Check sheet for the modelled part. Datum: model origin and axes. Units: mm. Give positions to 0.01 mm unless a question says otherwise; leave off trailing zeros. Write each loop counter-clockwise with the first axis right and the second up, starting at its lowest first coordinate (ties: lowest second). Pieces come first, ordered by that corner, then holes. Notation, with made-up numbers: (81.5, 11) -> (137.5, 11) arc R7 ccw to (137.5, 23) -> close; hole circle Ø9 at (70, 79). An arc over 180 degrees is marked (long way). Answer as a JSON object with one key per item and string values.
from build123d import *

# Parameters (mm, degrees)
CHAMFER1_SIZE = 0.2
CHAMFER2_SIZE = 0.2
CHAMFER3_SIZE = 0.5
CHAMFER4_SIZE = 0.5
FILLET2_R     = 0.2


with BuildPart() as part:
    # Sketch1 → Revolve1 (revolve)
    with BuildSketch(Plane.XY, mode=Mode.PRIVATE) as revolve1_sk:
        Polygon((0, 0), (117, 0), (117, 1.5), (112, 1.5), (112, 3), (3, 3), (3, 2.5), (0, 2.5), align=None)
    revolve(revolve1_sk.sketch.rotate(Axis((0, 0, 0), (1, 0, 0)), 90), axis=Axis((0, 0, 0), (1, 0, 0)))

    # Chamfer1
    chamfer1_edges = [part.edges().sort_by_distance(p)[0] for p in [
        (112, 0, -3),
    ]]
    chamfer(chamfer1_edges, length=CHAMFER1_SIZE)

    # Chamfer2
    chamfer2_edges = [part.edges().sort_by_distance(p)[0] for p in [
        (3, 0, -3),
    ]]
    chamfer(chamfer2_edges, length=CHAMFER2_SIZE)

    # Chamfer3
    chamfer3_edges = [part.edges().sort_by_distance(p)[0] for p in [
        (0, 0, -2.5),
    ]]
    chamfer(chamfer3_edges, length=CHAMFER3_SIZE)

    # Chamfer4
    chamfer4_edges = [part.edges().sort_by_distance(p)[0] for p in [
        (117, 0, -1.5),
    ]]
    chamfer(chamfer4_edges, length=CHAMFER4_SIZE)

    # Fillet2
    fillet2_edges = [part.edges().sort_by_distance(p)[0] for p in [
        (112, 0, -1.5),
    ]]
    fillet(fillet2_edges, radius=FILLET2_R)


solid = part.part
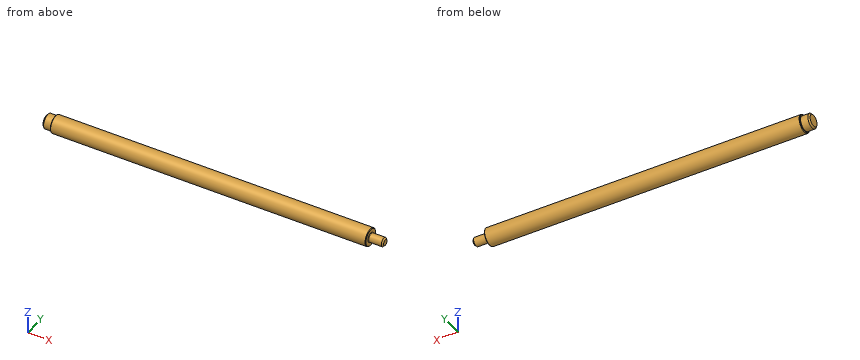
1. Sectioned sample at A-A, the plane z = 0. Enter the section's corners in (x, y).
Determined:
{"outline": "(0, -2) -> (0.5, -2.5) -> (3, -2.5) -> (3, -2.8) -> (3.2, -3) -> (111.8, -3) -> (112, -2.8) -> (112, -1.7) arc R0.2 cw to (112.2, -1.5) -> (116.5, -1.5) -> (117, -1) -> (117, 1) -> (116.5, 1.5) -> (112.2, 1.5) arc R0.2 cw to (112, 1.7) -> (112, 2.8) -> (111.8, 3) -> (3.2, 3) -> (3, 2.8) -> (3, 2.5) -> (0.5, 2.5) -> (0, 2) -> close"}
2. Sectioned sample at C-C, the plane x = 12.5. Enter the section's corners in (y, z), plus the area to 3 significant figures.
Determined:
{"outline": "circle Ø6 at (0, 0)", "area": "28.3 mm^2"}
3. Scan lines: L1, parallel to Y at x = 51.5, z = -1.1; L2, parallel to X at y = 0.2, z = -1.8; L3, parallel to Y at x = 54, z = 0.35. Record each from-to range of solid material in increasing order. Write a range as [from, to].
Determined:
{"L1": "[-2.79, 2.79]", "L2": "[0, 112]", "L3": "[-2.98, 2.98]"}
